```python
from build123d import *

# Parameters (mm, degrees)
SKETCH1_W           = 8
SKETCH1_H           = 5.461
BOSS_EXTRUDE1_DEPTH = 4.7625
CHAMFER1_SIZE       = 5.08


with BuildPart() as part:
    # Sketch1 → Boss-Extrude1 (new body)
    with BuildSketch(Plane.XY):
        Polygon((43.598645263, 119.489), (0, 119.489), (0, 111.361), (5, 111.361), (5, 105.9), (0, 105.9), (0, 73.261), (5, 73.261), (5, 67.8), (0, 67.8), (0, 43.561), (5, 43.561), (5, 38.1), (0, 38.1), (0, -38.1), (5, -38.1), (5, -43.561), (0, -43.561), (0, -67.8), (5, -67.8), (5, -73.261), (0, -73.261), (0, -105.9), (5, -105.9), (5, -111.361), (0, -111.361), (0, -119.489), (43.598645263, -119.489), (43.598645263, -111.361), (38.598645263, -111.361), (38.598645263, -105.9), (43.598645263, -105.9), (43.598645263, -73.261), (38.598645263, -73.261), (38.598645263, -67.8), (43.598645263, -67.8), (43.598645263, -43.561), (38.598645263, -43.561), (38.598645263, -38.1), (43.598645263, -38.1), (43.598645263, 38.1), (38.598645263, 38.1), (38.598645263, 43.561), (43.598645263, 43.561), (43.598645263, 67.8), (38.598645263, 67.8), (38.598645263, 73.261), (43.598645263, 73.261), (43.598645263, 105.9), (38.598645263, 105.9), (38.598645263, 111.361), (43.598645263, 111.361), align=None)
        with Locations((21.799322631, 108.6305)):
            Rectangle(SKETCH1_W, SKETCH1_H, mode=Mode.SUBTRACT)
        with Locations((21.799322631, 70.5305)):
            Rectangle(SKETCH1_W, SKETCH1_H, mode=Mode.SUBTRACT)
        with Locations((21.799322631, 40.8305)):
            Rectangle(SKETCH1_W, SKETCH1_H, mode=Mode.SUBTRACT)
        with Locations((21.799322631, -40.8305)):
            Rectangle(SKETCH1_W, SKETCH1_H, mode=Mode.SUBTRACT)
        with Locations((21.799322631, -70.5305)):
            Rectangle(SKETCH1_W, SKETCH1_H, mode=Mode.SUBTRACT)
        with Locations((21.799322631, -108.6305)):
            Rectangle(SKETCH1_W, SKETCH1_H, mode=Mode.SUBTRACT)
    extrude(amount=BOSS_EXTRUDE1_DEPTH)

    # Chamfer1
    chamfer1_edges = [part.edges().sort_by_distance(p)[0] for p in [
        (43.598645263, -119.489, 2.38125),
        (0, -119.489, 2.38125),
        (0, 119.489, 2.38125),
        (43.598645263, 119.489, 2.38125),
    ]]
    chamfer(chamfer1_edges, length=CHAMFER1_SIZE)


solid = part.part
```
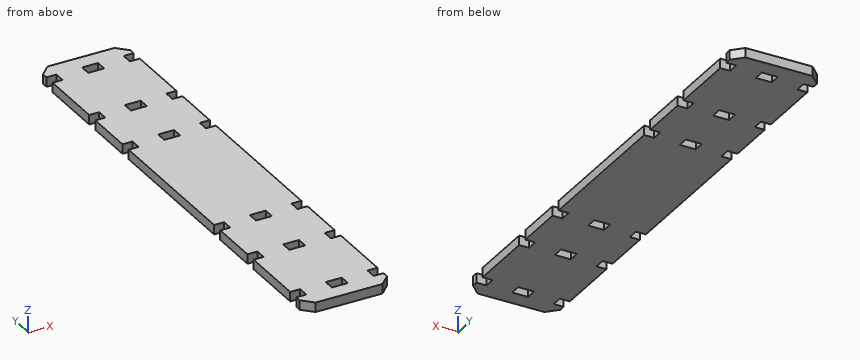
Can you work these out from the model? Positions are in its coordinate system, mm. Give positions to 0.01 mm unless a question says otherwise; leave off trailing zeros. Loops run counter-clockwise (first coordinate to the right, second up) from the corner with the lowest first, then second, coordinate; pieces in that order, holes last. Notation, with made-up numbers: M 62,-4 L 95,-4 A18 ccw 95,2 Z; hole C -5.5,67 d6. An arc over 180 degrees is marked long. Use one line per item in the form item = value. Start each with the question number.
(1) I want a section at A-A, the plane y = 41. Write out the boundary of the cut face in (x, z), and give its area (3 significant figures).
(2) Please list where this line runs through material, in increasing order: line 1 (X direction, y = 71, z = 0.95).
(3) I'm going to push flat-ended pins straight in: P1, Ø1.4, axis at x = 2, z = 3, coming from the +Y side; P2, Ø2.5, axis at x = 2.5, z = 1.5, coming from the -Y side; P3, Ø2.5, axis at x = 40, z = 2.5, coming from the -Y side. Where does each tip first touch, or does it pass through?
(4) I want a section at B-B, the plane z = 2.95. State how many separate pieces and enclosed holes the cut face has, and give its area (3 significant figures).
Worked out:
q1.outline = M 5,0 L 17.8,0 L 17.8,4.76 L 5,4.76 Z; M 25.8,0 L 38.6,0 L 38.6,4.76 L 25.8,4.76 Z
q1.area = 122 mm²
q2.line_1 = 5 to 17.8, 25.8 to 38.6
q3.P1 = 117.11
q3.P2 = -118.16
q3.P3 = -119.26
q4.separate_pieces = 1
q4.enclosed_holes = 6
q4.area = 9,780 mm²
